from build123d import *

# Parameters (mm, degrees)
SKETCH1_R           = 1.35
BOSS_EXTRUDE1_DEPTH = 3
SKETCH2_R           = 2.5
CUT_EXTRUDE1_DEPTH  = 1.7
CHAMFER1_SIZE       = 1.2


with BuildPart() as part:
    # Sketch1 → Boss-Extrude1 (new body)
    with BuildSketch(Plane(origin=(0, 0, 0), x_dir=(1, 0, 0), z_dir=(0, 1, 0))):
        with BuildLine():
            Line((134.161534911, 59.43281878), (-37.78892646, 59.059864213))
            add(Edge.make_bspline(
                [(-37.78892646, 59.059864213), (-39.260373987, 59.056672695), (-40.726264192, 58.873631016), (-42.864744181, 58.335544499), (-43.56477321, 58.113464931), (-44.928422176, 57.586554564), (-45.593707509, 57.281316649), (-46.242490458, 56.934388883)],
                knots=[0, 0, 0, 0, 0.5, 0.5, 0.75, 0.75, 1, 1, 1, 1], degree=3))
            Line((-46.242490458, 56.934388883), (-119.214433491, 17.913645156))
            add(Edge.make_bspline(
                [(-119.214433491, 17.913645156), (-119.371714153, 17.829541484), (-119.518068848, 17.731347507), (-119.789747392, 17.507837833), (-119.916274323, 17.380912308), (-120.139852202, 17.106706149), (-120.236961752, 16.960118582), (-120.402064762, 16.648131274), (-120.469932783, 16.481746722), (-120.570167022, 16.144162456), (-120.603591555, 15.971345529), (-120.63629684, 15.61747918), (-120.635015098, 15.439777034), (-120.598507798, 15.090011023), (-120.562994402, 14.91558609), (-120.458204018, 14.575953541), (-120.389758062, 14.412551149), (-120.305177563, 14.255596117)],
                knots=[0, 0, 0, 0, 0.125, 0.125, 0.25, 0.25, 0.375, 0.375, 0.5, 0.5, 0.625, 0.625, 0.75, 0.75, 0.875, 0.875, 1, 1, 1, 1], degree=3))
            Line((-120.305177563, 14.255596117), (-89.830246023, -42.296373733))
            add(Edge.make_bspline(
                [(-89.830246023, -42.296373733), (-88.375146858, -44.996584036), (-87.11307972, -47.796479497), (-84.994631409, -53.553509169), (-84.143686828, -56.492865486), (-83.501659246, -59.49224952)],
                knots=[0, 0, 0, 0, 0.5, 0.5, 1, 1, 1, 1], degree=3))
            add(Edge.make_bspline(
                [(-83.501659246, -59.49224952), (-83.207913745, -60.86455126), (-82.798283173, -62.200751268), (-82.010871212, -64.151167066), (-81.721235964, -64.787858992), (-81.092273153, -66.026650793), (-80.072714097, -67.836944856), (-78.830441112, -69.507100935), (-76.968111095, -71.604375976), (-75.952258591, -72.567256281), (-74.854523467, -73.441463587)],
                knots=[0, 0, 0, 0, 0.25, 0.25, 0.375, 0.375, 0.5, 0.75, 0.75, 1, 1, 1, 1], degree=3))
            Line((-74.854523467, -73.441463587), (-51.539950225, -92.008574916))
            add(Edge.make_bspline(
                [(-51.539950225, -92.008574916), (-51.390987712, -92.127204734), (-51.232429983, -92.228435853), (-50.896866499, -92.397446873), (-50.717603486, -92.465650862), (-50.353220614, -92.562423021), (-50.167823032, -92.591707222), (-49.790547653, -92.611667192), (-49.599550596, -92.601753163), (-49.228628709, -92.543472736), (-49.045331803, -92.494850179), (-48.690867071, -92.359239211), (-48.52347813, -92.273968718), (-48.207935535, -92.069298914), (-48.058689904, -91.948371285), (-47.792751324, -91.681532762), (-47.674455998, -91.534984666), (-47.571321486, -91.374872149)],
                knots=[0, 0, 0, 0, 0.125, 0.125, 0.25, 0.25, 0.375, 0.375, 0.5, 0.5, 0.625, 0.625, 0.75, 0.75, 0.875, 0.875, 1, 1, 1, 1], degree=3))
            add(Edge.make_bspline(
                [(-47.571321486, -91.374872149), (-46.153036919, -89.173037798), (-44.608917961, -87.076393648), (-41.274741201, -83.088695854), (-39.484564632, -81.197538353), (-35.653029438, -77.626010441), (-33.646571022, -75.978127616), (-29.459465947, -72.9471878), (-27.278793496, -71.564170023), (-23.876425351, -69.689354772), (-22.720413119, -69.097695924), (-20.363479447, -67.982655618), (-19.159804228, -67.458437514), (-15.529771039, -66.009292146), (-10.611085077, -64.391548948), (-5.539520445, -63.385094495), (-1.677546074, -62.863371081), (-0.379428844, -62.728223796), (2.232268288, -62.538422964), (3.539898616, -62.484137167), (4.849299501, -62.470210553)],
                knots=[0, 0, 0, 0, 0.125, 0.125, 0.25, 0.25, 0.375, 0.375, 0.5, 0.5, 0.5625, 0.5625, 0.625, 0.625, 0.75, 0.875, 0.875, 0.9375, 0.9375, 1, 1, 1, 1], degree=3))
            Line((4.849299501, -62.470210553), (134.990197336, -61.08604937))
            add(Edge.make_bspline(
                [(134.990197336, -61.08604937), (135.167346788, -61.084165224), (135.341361144, -61.064937541), (135.683502878, -60.993915065), (135.853395352, -60.941308848), (136.17721181, -60.80435926), (136.330630434, -60.720947254), (136.620639449, -60.524514457), (136.757918371, -60.410322016), (137.003647924, -60.161160095), (137.113655434, -60.025415528), (137.307455362, -59.731164559), (137.38973844, -59.574273341), (137.586799708, -59.088862557), (137.655136112, -58.736369262), (137.652832045, -58.382163441)],
                knots=[0, 0, 0, 0, 0.125, 0.125, 0.25, 0.25, 0.375, 0.375, 0.5, 0.5, 0.625, 0.625, 0.75, 0.75, 1, 1, 1, 1], degree=3))
            Line((137.652832045, -58.382163441), (136.904111112, 56.7188799))
            add(Edge.make_bspline(
                [(136.904111112, 56.7188799), (136.902940109, 56.898896811), (136.883766744, 57.075714075), (136.811945539, 57.42339902), (136.758448028, 57.596083274), (136.619240417, 57.924944469), (136.534418559, 58.080811621), (136.334727886, 58.375638017), (136.21883457, 58.51509664), (135.966139935, 58.765058133), (135.828467671, 58.877195989), (135.529967832, 59.07521276), (135.371179474, 59.159347789), (134.879114282, 59.361936915), (134.521405548, 59.433599309), (134.161534911, 59.43281878)],
                knots=[0, 0, 0, 0, 0.125, 0.125, 0.25, 0.25, 0.375, 0.375, 0.5, 0.5, 0.625, 0.625, 0.75, 0.75, 1, 1, 1, 1], degree=3))
        make_face()
        with Locations(Location((129.627717634, 51.726368816, 0), (0, 0, 270))):
            Circle(SKETCH1_R, mode=Mode.SUBTRACT)
        with Locations(Location((-31.164469896, 51.377616083, 0), (0, 0, 270))):
            Circle(SKETCH1_R, mode=Mode.SUBTRACT)
        with Locations(Location((-111.171184663, 13.369593003, 0), (0, 0, 270))):
            Circle(SKETCH1_R, mode=Mode.SUBTRACT)
        with Locations(Location((-50.65856493, -83.119927605, 0), (0, 0, 270))):
            Circle(SKETCH1_R, mode=Mode.SUBTRACT)
        with Locations(Location((4.947352904, -55.127624349, 0), (0, 0, 270))):
            Circle(SKETCH1_R, mode=Mode.SUBTRACT)
        with Locations(Location((130.314118933, -53.794240193, 0), (0, 0, 270))):
            Circle(SKETCH1_R, mode=Mode.SUBTRACT)
    extrude(amount=-BOSS_EXTRUDE1_DEPTH)

    # Sketch2 → Cut-Extrude1 (cut)
    with BuildSketch(Plane.XZ.offset(3)):
        with Locations(Location((-50.65856493, 83.119927605, 0), (0, 0, 270))):
            Circle(SKETCH2_R)
        with Locations(Location((4.947352904, 55.127624349, 0), (0, 0, 270))):
            Circle(SKETCH2_R)
        with Locations(Location((130.314118933, 53.794240193, 0), (0, 0, 270))):
            Circle(SKETCH2_R)
        with Locations(Location((129.627717634, -51.726368816, 0), (0, 0, 270))):
            Circle(SKETCH2_R)
        with Locations(Location((-31.164469896, -51.377616083, 0), (0, 0, 270))):
            Circle(SKETCH2_R)
        with Locations(Location((-111.171184663, -13.369593003, 0), (0, 0, 270))):
            Circle(SKETCH2_R)
    extrude(amount=-CUT_EXTRUDE1_DEPTH, mode=Mode.SUBTRACT)

    # Chamfer1
    # the kernel refuses this chamfer: 1.2 mm, written as the material it adds along each edge
    with BuildSketch(Plane(origin=(129.627717634, -1.3, -51.726368816), x_dir=(0, 0, -1), z_dir=(-1, 0, 0))) as chamfer1_piece_1_section:
        Polygon((2.5, CHAMFER1_SIZE), (2.5 - CHAMFER1_SIZE, 0), (2.5, 0), align=None)
    chamfer1_piece_1 = revolve(axis=Axis((129.627717634, -1.3, -51.726368816), (0, -1, 0)), mode=Mode.PRIVATE)
    chamfer1_piece_1 = chamfer1_piece_1 - Plane(origin=(129.627717634, -1.926520071, -51.726368816), x_dir=(0, 0, 1), z_dir=(0, 1, 0)) * Cylinder(1.35, 10, mode=Mode.PRIVATE)
    add(chamfer1_piece_1)
    with BuildSketch(Plane(origin=(130.314118933, -1.3, 53.794240193), x_dir=(0, 0, -1), z_dir=(-1, 0, 0))) as chamfer1_piece_2_section:
        Polygon((2.5, CHAMFER1_SIZE), (2.5 - CHAMFER1_SIZE, 0), (2.5, 0), align=None)
    chamfer1_piece_2 = revolve(axis=Axis((130.314118933, -1.3, 53.794240193), (0, -1, 0)), mode=Mode.PRIVATE)
    chamfer1_piece_2 = chamfer1_piece_2 - Plane(origin=(130.314118933, -1.926520071, 53.794240193), x_dir=(0, 0, 1), z_dir=(0, 1, 0)) * Cylinder(1.35, 10, mode=Mode.PRIVATE)
    add(chamfer1_piece_2)
    with BuildSketch(Plane(origin=(4.947352904, -1.3, 55.127624349), x_dir=(0, 0, -1), z_dir=(-1, 0, 0))) as chamfer1_piece_3_section:
        Polygon((2.5, CHAMFER1_SIZE), (2.5 - CHAMFER1_SIZE, 0), (2.5, 0), align=None)
    chamfer1_piece_3 = revolve(axis=Axis((4.947352904, -1.3, 55.127624349), (0, -1, 0)), mode=Mode.PRIVATE)
    chamfer1_piece_3 = chamfer1_piece_3 - Plane(origin=(4.947352904, -1.926520071, 55.127624349), x_dir=(0, 0, 1), z_dir=(0, 1, 0)) * Cylinder(1.35, 11, mode=Mode.PRIVATE)
    add(chamfer1_piece_3)
    with BuildSketch(Plane(origin=(-50.65856493, -1.3, 83.119927605), x_dir=(0, 0, -1), z_dir=(-1, 0, 0))) as chamfer1_piece_4_section:
        Polygon((2.5, CHAMFER1_SIZE), (2.5 - CHAMFER1_SIZE, 0), (2.5, 0), align=None)
    chamfer1_piece_4 = revolve(axis=Axis((-50.65856493, -1.3, 83.119927605), (0, -1, 0)), mode=Mode.PRIVATE)
    chamfer1_piece_4 = chamfer1_piece_4 - Plane(origin=(-50.65856493, -1.926520071, 83.119927605), x_dir=(0, 0, 1), z_dir=(0, 1, 0)) * Cylinder(1.35, 10, mode=Mode.PRIVATE)
    add(chamfer1_piece_4)
    with BuildSketch(Plane(origin=(-111.171184663, -1.3, -13.369593003), x_dir=(0, 0, -1), z_dir=(-1, 0, 0))) as chamfer1_piece_5_section:
        Polygon((2.5, CHAMFER1_SIZE), (2.5 - CHAMFER1_SIZE, 0), (2.5, 0), align=None)
    chamfer1_piece_5 = revolve(axis=Axis((-111.171184663, -1.3, -13.369593003), (0, -1, 0)), mode=Mode.PRIVATE)
    chamfer1_piece_5 = chamfer1_piece_5 - Plane(origin=(-111.171184663, -1.926520071, -13.369593003), x_dir=(0, 0, 1), z_dir=(0, 1, 0)) * Cylinder(1.35, 10, mode=Mode.PRIVATE)
    add(chamfer1_piece_5)
    with BuildSketch(Plane(origin=(-31.164469896, -1.3, -51.377616083), x_dir=(0, 0, -1), z_dir=(-1, 0, 0))) as chamfer1_piece_6_section:
        Polygon((2.5, CHAMFER1_SIZE), (2.5 - CHAMFER1_SIZE, 0), (2.5, 0), align=None)
    chamfer1_piece_6 = revolve(axis=Axis((-31.164469896, -1.3, -51.377616083), (0, -1, 0)), mode=Mode.PRIVATE)
    chamfer1_piece_6 = chamfer1_piece_6 - Plane(origin=(-31.164469896, -1.926520071, -51.377616083), x_dir=(0, 0, 1), z_dir=(0, 1, 0)) * Cylinder(1.35, 10, mode=Mode.PRIVATE)
    add(chamfer1_piece_6)


solid = part.part
The listing builds one solid part. Answer for the finished solid, in the listing's coordinates (mm). A direction names the side the tool comes from. Coordinates: 2 decimals unless noted, no trailing zeros. Order: outer loops, then holes, each group sorted by start corner. A loop starts at its lowest first (then second) coordinate and runs counter-clockwise, first axis right, second up.
Q1. Consider line 1 (X direction, y = -2.45, z = 82.5); line 2 (Z direction, x = -5, y = -2.3); line 3 (Z direction, x = 30, y = -1.5). Determine where each line is inside the solid, lowest interval first.
Q2. For a pull along Z with two mould halves and no side action, classify faces 1 (the face through (-63.36, -1.479, 82.595)), 2 (the face through (-82.218, -1.479, -37.697)), 3 (the face through (-113.4, -2.8, -14.5)) as pulls with the +Z half, pulls with the -Z half, needs draft (parallel to the pull), parting line crosses it, or undercut.
Q3. A cutting plane is placed at B-B, the plane z = 15. Write down the section's boundary in (x, y).
Q4. A cutting plane is placed at A-A, the plane y = -1.9. State how many separate pieces and enclosed holes the cut face has, and give its area (3 significant figures).
Q5. A cutting plane is placed at C-C, the plane x = 89. Write down the section's boundary in (y, z).
Q6. Given P1, Ø2, axis at x = -111.17, z = -13.37, coming from the +Y side; P2, Ø3, axis at x = 129.63, z = -51.73, coming from the -Y side, each flat-ended and moving along its own axis, determine where each tip first touches the part or whether it passes through.
Q7. Which of the six approach directions +Z, -Z, +X, -X, +Y, -Y give full straight-line access (tool end or side, diameter ignored) to faces 4 (the face through (7, 0, -1)), 5 (the face through (132.42, -2.75, 52.45))?
Answers follow:
1. line 1: x = -63.48 to -53.03, -48.29 to -40.66
1. line 2: z = -59.13 to 63.35
1. line 3: z = -59.21 to 62.2
2. face 1: pulls with the +Z half
2. face 2: pulls with the -Z half
2. face 3: undercut
3. outline: (-104.54, -3) - (137.37, -3) - (137.37, 0) - (-104.54, 0) - close
4. separate pieces: 1
4. enclosed holes: 6
4. area: 29,100 mm2
5. outline: (-3, -59.33) - (0, -59.33) - (0, 61.58) - (-3, 61.58) - close
6. P1: passes through
6. P2: stops at y = -1.5
7. face 4: +Z, -Z, +X, -X, +Y
7. face 5: -Y
